from build123d import *

# Parameters (mm, degrees)
F0_W     = 12.7
F0_H     = 12.7
F0_W_2   = 6.35
F0_H_2   = 17.78
F1_DEPTH = 12.7
F2_DEPTH = 15.24


with BuildPart() as f1:
    # F0 (on Front) → F1 (new body)
    with BuildSketch(Plane.XZ):
        with Locations((-20.219863, -11.348728)):
            Rectangle(F0_W, F0_H)
        with Locations((38.200137, -11.348728)):
            Rectangle(F0_W, F0_H)
        Polygon((2.640137, -4.998728), (-13.869863, -4.998728), (-13.869863, -17.698728), (31.850137, -17.698728), (31.850137, -4.998728), (15.340137, -4.998728), align=None)
        Polygon((8.990137, 21.671272), (2.640137, 21.671272), (2.640137, -4.998728), (15.340137, -4.998728), (15.340137, 21.671272), align=None)
        with Locations((12.165137, 30.561272)):
            Rectangle(F0_W_2, F0_H_2)
        with Locations((5.815137, 30.561272)):
            Rectangle(F0_W_2, F0_H_2)
        Polygon((2.640137, 49.611272), (2.640137, 39.451272), (8.990137, 39.451272), (15.340137, 39.451272), (15.340137, 49.611272), align=None)
    extrude(amount=F1_DEPTH)

    # F0 (on Front) → F2 (join)
    with BuildSketch(Plane.XZ):
        Polygon((2.640137, 49.611272), (2.640137, 39.451272), (8.990137, 39.451272), (15.340137, 39.451272), (15.340137, 49.611272), align=None)
        with Locations((-20.219863, -11.348728)):
            Rectangle(F0_W, F0_H)
        with Locations((38.200137, -11.348728)):
            Rectangle(F0_W, F0_H)
    extrude(amount=-F2_DEPTH)


solid = f1.part
For this review, take the finished solid that the model builds, in its own axes (mm). A direction names the side the tool comes from. Give positions to 0.01 mm unless a question says otherwise; leave off trailing zeros. Order: outer loops, then holes, each group sorted by start corner. A loop starts at its lowest first (then second) coordinate and runs counter-clockwise, first axis right, second up. Notation, with made-up numbers: (5.25, 18) - (58.25, 18) arc R34 ccw to (58.25, 51) - close; hole circle Ø10 at (-2, 13). An arc over 180 degrees is marked (long way). Answer as a JSON object with one key per item and string values. Group by question number.
Item 1: Machinability: for faces 4 (the flat face through (2.64, -5, 29)), 5 (the flat face through (-13.87, 8, -11)), 6 (the flat face through (9, 8, 39.451)), 7 (the flat face through (33, -2, -4.999)), which of the approach directions +Z, -Z, +X, -X, +Y, -Y give a long, thin tool a straight path to every point of the face, cutting with its end or side? Answer none if there is none.
Item 2: Draft analysis for pull direction X (two halves, no side actions). For faces 1 (the flat face through (15.34, -5, 28)), 2 (the flat face through (9, 1, 49.611)), 3 (the flat face through (9, 0, 5)), state which applies: pulls with the +X half, pulls with the -X half, needs draft (parallel to the pull), parting line crosses it, or undercut.
Item 3: Wall thickness on line 1 along X through (y, z) = (5.75, -9); line 2 along X through (y, z) = (-0.5, 21); line 3 along Z through (x, y) = (-18.5, -5): over which ranges is each line inside the solid? List them lowest first.
Item 4: Take a section at C-C on z = -10. Give the boundary of the cut face in (x, y).
Item 5: Take a section at D-D on x = 14. Give the boundary of the cut face in (y, z), and give its area (3 significant figures).
Item 6: Clearance check with flat-ended pins moving along their axes: pin 1 Ø12 at (x, z) = (3.5, -2) entering from +Y; pin 2 Ø12 at (y, z) = (7.5, 36.5) entering from +X; pin 3 Ø12 at (x, y) = (-17, -8) entering from +Z. State where each tip first meets the part, or that it passes through.
Item 7: Take a section at A-A on y = 11.5. Give the boundary of the cut face in (x, z).
Item 8: Take a section at B-B on y = -6.5. Give the boundary of the cut face in (x, z).
Reported:
{
 "1": {"face 4": "+Z, -X, +Y, -Y", "face 5": "+Z, -Z, +Y", "face 6": "-Z, +X, -X, +Y", "face 7": "+Z, +X, +Y, -Y"},
 "2": {"face 1": "pulls with the +X half", "face 2": "needs draft", "face 3": "undercut"},
 "3": {"line 1": "-26.57 to -13.87, 31.85 to 44.55", "line 2": "2.64 to 15.34", "line 3": "-17.7 to -5"},
 "4": {"outline": "(-26.57, -12.7) - (44.55, -12.7) - (44.55, 15.24) - (31.85, 15.24) - (31.85, 0) - (-13.87, 0) - (-13.87, 15.24) - (-26.57, 15.24) - close"},
 "5": {"outline": "(-12.7, -17.7) - (0, -17.7) - (0, 39.45) - (15.24, 39.45) - (15.24, 49.61) - (-12.7, 49.61) - close", "area": "1,010 mm^2"},
 "6": {"pin 1": "y = 0", "pin 2": "x = 15.34", "pin 3": "z = -5"},
 "7": {"outline": "(-26.57, -17.7) - (-13.87, -17.7) - (-13.87, -5) - (-26.57, -5) - close; (2.64, 39.45) - (15.34, 39.45) - (15.34, 49.61) - (2.64, 49.61) - close; (31.85, -17.7) - (44.55, -17.7) - (44.55, -5) - (31.85, -5) - close"},
 "8": {"outline": "(-26.57, -17.7) - (44.55, -17.7) - (44.55, -5) - (15.34, -5) - (15.34, 49.61) - (2.64, 49.61) - (2.64, -5) - (-26.57, -5) - close"}
}
